```python
from build123d import *

# Parameters (mm, degrees)
SKETCH_1_W                = 85.09
SKETCH_1_H                = 66.675
EXTRUDE_1_DEPTH           = 1.6
SKETCH_2_W                = 15.24
SKETCH_2_H                = 20.32
EXTRUDE_2_DEPTH           = 19
SKETCH_3_W                = 15.24
SKETCH_3_H                = 20.32
EXTRUDE_3_DEPTH           = 19
HOLE_WIZARD_3_0_3_1_D     = 3
HOLE_WIZARD_3_0_3_1_DEPTH = 20.6
FILLET_1_R                = 3.81


with BuildPart() as part:
    # 草图1 → 凸台-拉伸1 (new body)
    with BuildSketch(Plane.XY.offset(1.6)):
        with Locations((42.545, 33.3375)):
            Rectangle(SKETCH_1_W, SKETCH_1_H)
    extrude(amount=-EXTRUDE_1_DEPTH)

    # 草图2 → 凸台-拉伸2 (add)
    with BuildSketch(Plane.XY.offset(1.6)):
        with Locations((57.15, 24.13)):
            Rectangle(SKETCH_2_W, SKETCH_2_H)
    extrude(amount=EXTRUDE_2_DEPTH)

    # 草图3 → 凸台-拉伸3 (add)
    with BuildSketch(Plane.XY.offset(1.6)):
        with Locations((27.94, 24.13)):
            Rectangle(SKETCH_3_W, SKETCH_3_H)
    extrude(amount=EXTRUDE_3_DEPTH)

    # Ø3.0 (3) 直径孔1
    with Locations(Plane(origin=(0, 0, 0), x_dir=(-1, 0, 0), z_dir=(0, 0, -1))):
        with Locations((-3.81, 62.865), (-3.81, 3.81), (-81.28, 3.81), (-81.28, 62.865)):
            Hole(HOLE_WIZARD_3_0_3_1_D / 2, depth=HOLE_WIZARD_3_0_3_1_DEPTH)

    # 圆角1
    fillet_1_edges = [part.edges().sort_by_distance(p)[0] for p in [
        (0, 0, 0.8),
        (0, 66.675, 0.8),
        (85.09, 66.675, 0.8),
        (85.09, 0, 0.8),
    ]]
    fillet(fillet_1_edges, radius=FILLET_1_R)


solid = part.part
```
Here's how the part is built. I have some questions about the finished solid (model axes, mm). A direction names the side the tool comes from. Give positions to 0.01 mm unless a question says otherwise; leave off trailing zeros. Order: outer loops, then holes, each group sorted by start corner. A loop starts at its lowest first (then second) coordinate and runs counter-clockwise, first axis right, second up. Notation, with made-up numbers: M -17,-8 L 36,-8 A34 cw 36,24 Z; hole C 82.25,32 d11. An arc over 180 degrees is marked long. Use a Markdown table: item, result. Add a question column.
1. Suppose I cut it at C-C (x = 61). List the corners of the cut face in (y, z) for me (3 decimals), and give its area (3 significant figures).
2. Suppose I cut it at A-A (z = 14.5). List the corners of the cut face in (x, y) for me, and give its area (3 significant figures).
3. Suppose I cut it at B-B (y = 16). List the corners of the cut face in (x, z) for me, and give its area (3 significant figures).
4. If we mould it in two halves opening along X, with no side actions, what happens to faces 5 (the flat face through (20.32, 24, 11)), 6 (the flat face through (42, 34, 0)), 7 (the cylindrical face through (80.09, 61.95, 0.81))? For each: +X half, -X half, draft (parallel to the pull), parting line (faces both ways), or undercut.
5. On a 3-axis mill with a long thin cutter (end or side, diameter ignored), from which of +Z, -Z, +X, -X, +Y, -Y can I reach the whole of each face in a straight line? I mean faces 1 (the flat face through (35.56, 24, 11)), 2 (the flat face through (57, 34.29, 11)), 3 (the flat face through (57, 13.97, 11)), 4 (the cylindrical face through (4.616, 5.075, 0.811)). Say none if no direction works.
6. For pin 1 Ø2 at (x, y) = (41, 48) entering from +Z; pin 2 Ø2 at (x, z) = (22, 4) entering from -Y; pin 3 Ø12 at (y, z) = (23, 8) entering from +X, each with a flat end and sliding along its axis, tell me the tip position at first contact or that it passes through.
7. Suppose I cut it at D-D (x = 18). List the corners of the cut face in (y, z) for me (3 decimals), and give its area (3 significant figures).
8. I need wall thicknesses on probe 1 along Y at (x, z) = (81.28, 0.6) (3 decimals); probe 2 along X at (y, z) = (14, 13.25); probe 3 along Y at (x, z) = (62, 12.5). Which ranges of each line are inside material? Lowest first, please. Write a range as from..to.
Results list:
| question | item | result |
|---|---|---|
| 1 | outline | M 0,0 L 66.675,0 L 66.675,1.6 L 34.29,1.6 L 34.29,20.6 L 13.97,20.6 L 13.97,1.6 L 0,1.6 Z |
| 1 | area | 493 mm² |
| 2 | outline | M 20.32,13.97 L 35.56,13.97 L 35.56,34.29 L 20.32,34.29 Z; M 49.53,13.97 L 64.77,13.97 L 64.77,34.29 L 49.53,34.29 Z |
| 2 | area | 619 mm² |
| 3 | outline | M 0,0 L 85.09,0 L 85.09,1.6 L 64.77,1.6 L 64.77,20.6 L 49.53,20.6 L 49.53,1.6 L 35.56,1.6 L 35.56,20.6 L 20.32,20.6 L 20.32,1.6 L 0,1.6 Z |
| 3 | area | 715 mm² |
| 4 | face 5 | -X half |
| 4 | face 6 | draft |
| 4 | face 7 | undercut |
| 5 | face 1 | +Z, +Y, -Y |
| 5 | face 2 | +Z, +X, -X, +Y |
| 5 | face 3 | +Z, +X, -X, -Y |
| 5 | face 4 | +Z, -Z |
| 6 | pin 1 | stops at z = 1.6 |
| 6 | pin 2 | stops at y = 13.97 |
| 6 | pin 3 | stops at x = 64.77 |
| 7 | outline | M 0,0 L 66.675,0 L 66.675,1.6 L 0,1.6 Z |
| 7 | area | 107 mm² |
| 8 | probe 1 | y = 0..2.31, 5.31..61.365, 64.365..66.675 |
| 8 | probe 2 | x = 20.32..35.56, 49.53..64.77 |
| 8 | probe 3 | y = 13.97..34.29 |
